```python
from build123d import *

# Parameters (mm, degrees)
F0_R     = 12.7
F2_R     = 25.4
F3_DEPTH = 12.7
F4_R     = 3.175
F5_DEPTH = 25.4


with BuildPart() as f1:
    # F0 (on Top) → F1 (revolve)
    with BuildSketch(Plane.XY):
        with Locations((0, 25.4)):
            Circle(F0_R)
    revolve(axis=Axis((2.317362465, 0, 0), (1, 0, 0)))

    # F2 (on Right) → F3 (join, symmetric)
    with BuildSketch(Plane.YZ):
        Circle(F2_R)
    extrude(amount=F3_DEPTH, both=True)

    # F4 (on face) → F5 (cut)
    with BuildSketch(Plane.YZ.offset(12.7)):
        Circle(F4_R)
    extrude(amount=-F5_DEPTH, mode=Mode.SUBTRACT)


solid = f1.part
```
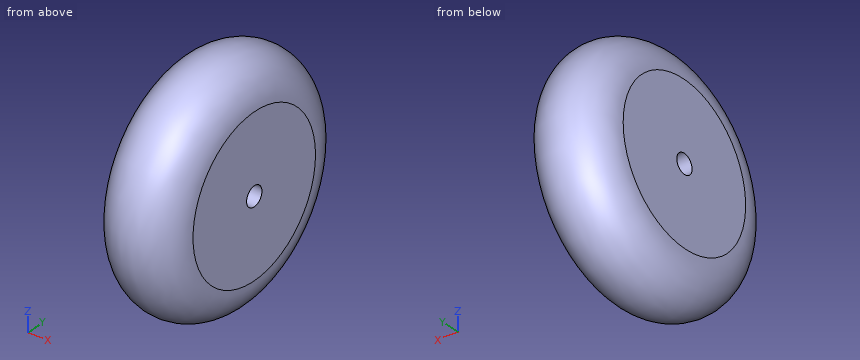
The model under review builds one solid part; all positions refer to its coordinate system, in mm. Give positions to 0.01 mm unless a question says otherwise; leave off trailing zeros. Write each loop counter-clockwise with the first axis right and the second up, starting at its lowest first coordinate (ties: lowest second). Pieces come first, ordered by that corner, then holes. Notation, with made-up numbers: (-37, 10) -> (16, 10) arc R11 cw to (16, 30) -> close; hole circle Ø11 at (-3, -7). An arc over 180 degrees is marked (long way). Answer in a Markdown table with one row per item.
1) Add section A-A on z = 0. State the section outline as (x, y) points (3 decimals).
Worked answers:
| item | result |
|---|---|
| outline | (-12.7, -25.4) arc R12.7 ccw to (12.7, -25.4) -> (12.7, -3.175) -> (-12.7, -3.175) -> close; (-12.7, 3.175) -> (12.7, 3.175) -> (12.7, 25.4) arc R12.7 ccw to (-12.7, 25.4) -> close |
2) Clearance check with flat-ended pins moving along their axes: P1, Ø4, axis at x = 9, y = -2, coming from the +Z side; P2, Ø10, axis at x = 5, z = -23, coming from the -Y side; P3, Ø1.5, axis at x = -3.5, y = -28.5, coming from the -Z side. State where each tip first meets the part, or that it passes through.
Worked answers:
| item | result |
|---|---|
| P1 | z = 35.95 |
| P2 | y = -32.94 |
| P3 | z = -25.44 |
3) Add section C-C on x = 9. State the section outline as (y, z) points (3 decimals).
Worked answers:
| item | result |
|---|---|
| outline | circle Ø68.721 at (0, 0); hole circle Ø6.35 at (0, 0) |
4) Add section D-D on x = 0.75. State the section outline as (y, z) points (3 decimals).
Worked answers:
| item | result |
|---|---|
| outline | circle Ø76.156 at (0, 0); hole circle Ø6.35 at (0, 0) |
5) For L1, parallel to X at y = -17.5, z = 19; L2, parallel to Z at x = 7.75, y = 0 (3 decimals); L3, parallel to Y at x = 6.25, z = -2, list the stretches that pass through material, from the lowest coordinate up. Write a range as [from, to].
Worked answers:
| item | result |
|---|---|
| L1 | [-12.69, 12.69] |
| L2 | [-35.461, -3.175], [3.175, 35.461] |
| L3 | [-36.4, -2.47], [2.47, 36.4] |
